from build123d import *

# Parameters (mm, degrees)
SKETCH_4_R      = 4.5
SKETCH_4_R_2    = 1.8
EXTRUDE_1_DEPTH = 6


with BuildPart() as part:
    # 草图4 → 凸台-拉伸1 (new body)
    with BuildSketch(Plane(origin=(0, 0, 0), x_dir=(1, 0, 0), z_dir=(0, 1, 0))):
        with BuildLine():
            Line((136.46105702, 22.159664941), (136.46105702, 47.159664941))
            Line((136.46105702, 47.159664941), (35.46105702, 47.159664941))
            ThreePointArc((35.46105702, 47.159664941), (34.046843458, 46.573878503), (33.46105702, 45.159664941))
            Line((33.46105702, 45.159664941), (33.46105702, 44.159664941))
            ThreePointArc((33.46105702, 44.159664941), (32.875270583, 42.745451378), (31.46105702, 42.159664941))
            Line((31.46105702, 42.159664941), (28.46105702, 42.159664941))
            ThreePointArc((28.46105702, 42.159664941), (27.046843458, 42.745451378), (26.46105702, 44.159664941))
            Line((26.46105702, 44.159664941), (26.46105702, 49.744433688))
            Line((26.46105702, 49.744433688), (26.46105702, 50.159664941))
            ThreePointArc((26.46105702, 50.159664941), (25.875270583, 51.573878503), (24.46105702, 52.159664941))
            Line((24.46105702, 52.159664941), (-71.53894298, 52.159664941))
            ThreePointArc((-71.53894298, 52.159664941), (-72.953156542, 51.573878503), (-73.53894298, 50.159664941))
            Line((-73.53894298, 50.159664941), (-73.53894298, 14.159664941))
            ThreePointArc((-73.53894298, 14.159664941), (-72.953156542, 12.745451378), (-71.53894298, 12.159664941))
            Line((-71.53894298, 12.159664941), (24.46105702, 12.159664941))
            ThreePointArc((24.46105702, 12.159664941), (25.875270583, 12.745451378), (26.46105702, 14.159664941))
            Line((26.46105702, 14.159664941), (26.46105702, 20.171292313))
            ThreePointArc((26.46105702, 20.171292313), (27.04343788, 21.577284081), (28.449429648, 22.159664941))
            Line((28.449429648, 22.159664941), (31.46105702, 22.159664941))
            ThreePointArc((31.46105702, 22.159664941), (32.875270583, 21.573878503), (33.46105702, 20.159664941))
            Line((33.46105702, 20.159664941), (33.46105702, 14.159664941))
            ThreePointArc((33.46105702, 14.159664941), (34.046843458, 12.745451378), (35.46105702, 12.159664941))
            Line((35.46105702, 12.159664941), (136.46105702, 12.159664941))
            Line((136.46105702, 12.159664941), (136.46105702, 22.159664941))
        make_face()
        with Locations((59.46105702, 21.159664941)):
            Circle(SKETCH_4_R, mode=Mode.SUBTRACT)
        with Locations((127.46105702, 21.159664941)):
            Circle(SKETCH_4_R, mode=Mode.SUBTRACT)
        with Locations((82.46105702, 27.159664941)):
            Circle(SKETCH_4_R_2, mode=Mode.SUBTRACT)
        with Locations((59.46105702, 38.159664941)):
            Circle(SKETCH_4_R, mode=Mode.SUBTRACT)
        with Locations((127.46105702, 38.159664941)):
            Circle(SKETCH_4_R, mode=Mode.SUBTRACT)
        with Locations((82.46105702, 42.159664941)):
            Circle(SKETCH_4_R_2, mode=Mode.SUBTRACT)
    extrude(amount=EXTRUDE_1_DEPTH)


solid = part.part
Input: part model. Units: mm. Frame: model coordinates. A direction names the side the tool comes from. Give positions to 0.01 mm unless a question says otherwise; leave off trailing zeros. Write each loop counter-clockwise with the first axis right and the second up, starting at its lowest first coordinate (ties: lowest second). Pieces come first, ordered by that corner, then holes. Notation, with made-up numbers: M 32.5,18.25 L 75.5,18.25 A31 cw 75.5,52.25 Z; hole C -31.5,19 d7. An arc over 180 degrees is marked long. Write item = value, one per line. Start each with the question number.
1) First-contact query: pin 1 Ø3 at (x, y) = (57.5, 5) entering from -Z; pin 2 Ø1.5 at (x, y) = (30, 3) entering from -Z; pin 3 Ø3 at (x, z) = (82.46, -42.16) entering from +Y; pin 4 Ø2.5 at (x, y) = (30, 4) entering from +Z. Flat tips, straight axial feed; report the tip coordinate or a pass-through.
2) Draft query along X for faces 1 (the cylindrical face through (84.18, 2.96, -42.7)), 2 (the flat face through (136.461, 3, -29)), 3 (the flat face through (30, 6, -32)). Return one class per face: +X half, -X half, draft (parallel to the pull), parting line (faces both ways), or undercut.
3) Cut plane B-B on y = 4.35. Return the cut outline in (x, z).
4) Material intervals for line 1 along X through (y, z) = (2.5, -23); line 2 along X through (y, z) = (4.45, -35.5); line 3 along X through (y, z) = (2.35, -18.5), sorted ascending. Write a range as [from, to].
5) Reachability of faces 4 (the flat face through (87, 3, -47.16)), 5 (the flat face through (-73.539, 3, -32)), 6 (the flat face through (26.461, 3, -47)), 7 (the cylindrical face through (84.124, 2.958, -26.47)), 8 (the flat face through (33.461, 3, -17)) from +Z, -Z, +X, -X, +Y, -Y: full face, straight path, thin tool, end or side. Return the list, or none.
6) Cut plane A-A on x = 103.5. Return the cut outline in (y, z), then the cut area to 3 significant figures.
Solved:
q1.pin_1 = -47.16
q1.pin_2 = -42.16
q1.pin_3 = through
q1.pin_4 = -22.16
q2.face_1 = undercut
q2.face_2 = +X half
q2.face_3 = draft
q3.outline = M -73.54,-50.16 A2 ccw -71.54,-52.16 L 24.46,-52.16 A2 ccw 26.46,-50.16 L 26.46,-44.16 A2 cw 28.46,-42.16 L 31.46,-42.16 A2 cw 33.46,-44.16 L 33.46,-45.16 A2 ccw 35.46,-47.16 L 136.46,-47.16 L 136.46,-12.16 L 35.46,-12.16 A2 ccw 33.46,-14.16 L 33.46,-20.16 A2 cw 31.46,-22.16 L 28.45,-22.16 A1.99 cw 26.46,-20.17 L 26.46,-14.16 A2 ccw 24.46,-12.16 L -71.54,-12.16 A2 ccw -73.54,-14.16 Z; hole C 59.46,-38.16 d9; hole C 59.46,-21.16 d9; hole C 82.46,-42.16 d3.6; hole C 82.46,-27.16 d3.6; hole C 127.46,-38.16 d9; hole C 127.46,-21.16 d9
q4.line_1 = [-73.54, 55.35], [63.57, 123.35], [131.57, 136.46]
q4.line_2 = [-73.54, 55.83], [63.09, 123.83], [131.09, 136.46]
q4.line_3 = [-73.54, 26.46], [33.46, 55.83], [63.09, 123.83], [131.09, 136.46]
q5.face_4 = -Z, +X, +Y, -Y
q5.face_5 = +Z, -Z, -X, +Y, -Y
q5.face_6 = -Z, +Y, -Y
q5.face_7 = +Y, -Y
q5.face_8 = +Z, +Y, -Y
q6.outline = M 0,-47.16 L 6,-47.16 L 6,-12.16 L 0,-12.16 Z
q6.area = 210 mm2
